Solid Edge part; units mm, degrees
sketch "Sketch1" plane through (0, 0, 0) normal (0, 0, 1) x (1, 0, 0)
  line L0 (-3.5, -7) -> (3.5, -7)
  line L1 (3.5, -7) -> (3.5, 7)
  line L2 (3.5, 7) -> (-3.5, 7)
  line L3 (-3.5, 7) -> (-3.5, -7)
  dimension "D1" = 3.5
  dimension "D2" = 3.5
extrude "Protrusion1" add sketch "Sketch1" along normal blind 1.5
sketch "Sketch2" plane through (0, 0, 1.5) normal (0, 0, 1) x (1, 0, 0)
  line L0 (-3.5, 7) -> (3.5, 7)
  line L1 (3.5, 7) -> (3.5, 5)
  line L2 (3.5, 5) -> (-3.5, 5)
  line L3 (-3.5, 5) -> (-3.5, 7)
  line L4 (-3.5, -7) -> (3.5, -7)
  line L5 (3.5, -7) -> (3.5, -5)
  line L6 (3.5, -5) -> (-3.5, -5)
  line L7 (-3.5, -5) -> (-3.5, -7)
  dimension "D1" = 3.5
extrude "Extrusionsausprägung_2" add sketch "Sketch2" along normal blind 7
sketch "Sketch3" plane through (0, 0, 0) normal (0, 0, -1) x (0, -1, 0)
  line L0 (-7, 3.5) -> (7, 3.5)
  arc A0 (-7, 3.5) -> (7, 3.5) centre (0, 3.5) cw
extrude "Extrusionsausprägung_3" add sketch "Sketch3" against normal blind 1.5
sketch "Sketch4" plane through (0, 6, 8.5) normal (0, 0, 1) x (1, 0, 0)
  line L0 (-3.5, 1) -> (-3, 1)
  line L1 (-3, 1) -> (-3, -1)
  line L2 (-3, -1) -> (-3.5, -1)
  line L3 (-3.5, -1) -> (-3.5, 1)
  line L4 (3.5, 1) -> (3, 1)
  line L5 (3, 1) -> (3, -1)
  line L6 (3, -1) -> (3.5, -1)
  line L7 (3.5, -1) -> (3.5, 1)
  line L8 (-3.5, -11) -> (-3, -11)
  line L9 (-3, -11) -> (-3, -13)
  line L10 (-3, -13) -> (-3.5, -13)
  line L11 (-3.5, -13) -> (-3.5, -11)
  line L12 (3.5, -11) -> (3, -11)
  line L13 (3, -11) -> (3, -13)
  line L14 (3, -13) -> (3.5, -13)
  line L15 (3.5, -13) -> (3.5, -11)
  dimension "D1" = 3
extrude "Cutout1" cut sketch "Sketch4" against normal up to vertex (7 mm away)
chamfer "Fase_1" distance 1 angle 45 2 edges at (0, 5, 8.5) (0, -5, 8.5)
properties material "Nylon, allgemein"
Read the model definition and answer for the solid it produces. Units are mm, in the model's axes. A direction names the side the tool comes from. Round coordinates to 2 decimals unless told otherwise and drop trailing zeros. Order: outer loops, then holes, each group sorted by start corner. A loop starts at its lowest first (then second) coordinate and runs counter-clockwise, first axis right, second up.
1) The mould has two halves that part along Y. Classify faces 1 (the face through (-4, 0, 1.5)), 2 (the face through (0, 6.5, 8.5)), 3 (the face through (-10.5, -0.15, 0.74)): released by +Y, released by -Y, zero draft, split by the parting line, or undercut.
2) The part is cut by section C-C on z = 4. Write down the section's boundary in (x, y), plus the area to 3 significant figures.
3) Flat-ended cylindrical pins translate along their axes: pin 1 (1 mm diameter, centred on y = 5, z = 1.5, fed in from -X); pin 2 (2 mm diameter, centred on y = -6, z = 5.5, fed in from +X); pin 3 (2 mm diameter, centred on y = 2, z = 1.5, fed in from -X). Find the tip coordinate at first contact, or state that the pin passes through.
4) For faces 4 (the face through (3, 6, 5)), 5 (the face through (0, -5, 4)), 6 (the face through (-3, -6, 5)), determine the directions among +Z, -Z, +X, -X, +Y, -Y from which every point of the face is accessible in a straight line to the end or side of a thin tool.
5) The part is cut by section B-B on x = 2.75. Write down the section's boundary in (y, z).
6) The part is cut by section D-D on y = 0.25. Write down the section's boundary in (x, z).
7) Straight lines are drawn through the part: L1, parallel to Y at x = -0.5, z = 2.5; L2, parallel to Z at x = -2.25, y = -0.25; L3, parallel to X at y = 6.5, z = 3.5. For each, find the intervals that lie inside material, in ascending order.
8) The part is cut by section A-A on z = 8. Write down the section's boundary in (x, y), plus the area to 3 significant figures.
Resolved:
1. face 1: undercut
1. face 2: zero draft
1. face 3: split by the parting line
2. outline: (-3, -7) - (3, -7) - (3, -5) - (-3, -5) - close; (-3, 5) - (3, 5) - (3, 7) - (-3, 7) - close
2. area: 24.0 mm2
3. pin 1: stops at x = -8.86
3. pin 2: stops at x = 3
3. pin 3: stops at x = -10.43
4. face 4: +Z, +X, +Y, -Y
4. face 5: +Z, +X, -X
4. face 6: +Z, -X, +Y, -Y
5. outline: (-7, 0) - (7, 0) - (7, 8.5) - (6, 8.5) - (5, 7.5) - (5, 1.5) - (-5, 1.5) - (-5, 7.5) - (-6, 8.5) - (-7, 8.5) - close
6. outline: (-10.5, 0) - (3.5, 0) - (3.5, 1.5) - (-10.5, 1.5) - close
7. L1: y = -7 to -5, 5 to 7
7. L2: z = 0 to 1.5
7. L3: x = -3 to 3
8. outline: (-3, -7) - (3, -7) - (3, -5.5) - (-3, -5.5) - close; (-3, 5.5) - (3, 5.5) - (3, 7) - (-3, 7) - close
8. area: 18.0 mm2
